Source: CAD feature listing. Evaluate the final solid. Frame: model axes, mm. Face numbers are marked on the shaded views. Give positions to 0.01 mm unless a question says otherwise; leave off trailing zeros. Loops run counter-clockwise (first coordinate to the right, second up) from the corner with the lowest first, then second, coordinate; pieces in that order, holes last. Notation, with made-up numbers: M -17.75,-13 L 12.25,-13 A17 cw 12.25,19 Z; hole C 85.5,50.5 d2. An arc over 180 degrees is marked long. Answer in a Markdown table with one row per item.
```python
from build123d import *

# Parameters (mm, degrees)
SKETCH1_R           = 37
BOSS_EXTRUDE1_DEPTH = 3.158172797
SKETCH13_W          = 7.575673387
SKETCH13_H          = 3.158172797
SKETCH13_W_2        = 7.5
BOSS_EXTRUDE2_DEPTH = 60
CIRPATTERN1_COUNT   = 4
SKETCH2_R           = 35
SKETCH2_R_2         = 6.35
CUT_EXTRUDE1_DEPTH  = 1
SKETCH17_R          = 2
CUT_EXTRUDE2_DEPTH  = 10
SKETCH19_R          = 1.5
CUT_EXTRUDE3_DEPTH  = 10
CIRPATTERN2_COUNT   = 4


with BuildPart() as part:
    # Sketch1 → Boss-Extrude1 (new body)
    with BuildSketch(Plane(origin=(0, 0, 0), x_dir=(1, 0, 0), z_dir=(0, 1, 0))):
        Circle(SKETCH1_R)
    extrude(amount=BOSS_EXTRUDE1_DEPTH)

    # Sketch13 → Boss-Extrude2 (add)
    with BuildSketch(Plane.XY):
        with Locations((3.787836694, 1.579086399)):
            Rectangle(SKETCH13_W, SKETCH13_H)
        with Locations((-3.75, 1.579086399)):
            Rectangle(SKETCH13_W_2, SKETCH13_H)
    boss_extrude2 = extrude(amount=BOSS_EXTRUDE2_DEPTH)

    # CirPattern1: Boss-Extrude2 ×4 about axis
    cirpattern1_axis = Axis((0, 0, 0), (0, 1, 0))
    for i in range(1, CIRPATTERN1_COUNT):
        add(boss_extrude2.rotate(cirpattern1_axis, i * 360 / CIRPATTERN1_COUNT))

    # Sketch2 → Cut-Extrude1 (cut)
    with BuildSketch(Plane(origin=(0, 3.158172797, 0), x_dir=(1, 0, 0), z_dir=(0, 1, 0))):
        Circle(SKETCH2_R)
        Circle(SKETCH2_R_2, mode=Mode.SUBTRACT)
    extrude(amount=-CUT_EXTRUDE1_DEPTH, mode=Mode.SUBTRACT)

    # Sketch17 → Cut-Extrude2 (cut)
    with BuildSketch(Plane(origin=(0, 3.158172797, 0), x_dir=(1, 0, 0), z_dir=(0, 1, 0))):
        Circle(SKETCH17_R)
    extrude(amount=-CUT_EXTRUDE2_DEPTH, mode=Mode.SUBTRACT)

    # Sketch19 → Cut-Extrude3 (cut)
    with BuildSketch(Plane(origin=(0, 3.158172797, 0), x_dir=(1, 0, 0), z_dir=(0, 1, 0))):
        with Locations((0, 25)):
            Circle(SKETCH19_R)
    cut_extrude3 = extrude(amount=-CUT_EXTRUDE3_DEPTH, mode=Mode.SUBTRACT)

    # CirPattern2: Cut-Extrude3 ×4 about axis
    cirpattern2_axis = Axis((0, 0, 0), (0, 1, 0))
    for i in range(1, CIRPATTERN2_COUNT):
        add(cut_extrude3.rotate(cirpattern2_axis, i * 360 / CIRPATTERN2_COUNT), mode=Mode.SUBTRACT)


solid = part.part
```
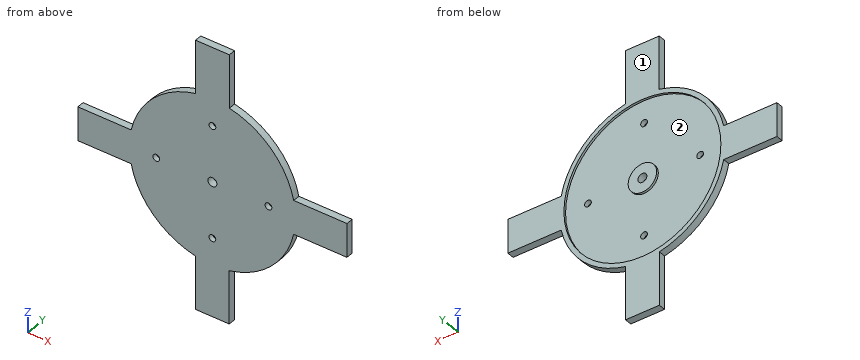
1) Pull-direction query (X, two-part tool) for the marked faces 1 and 2; classes: released by +X, released by -X, zero draft, split by the parting line, or undercut.
Reply:
| item | result |
|---|---|
| face 1 | zero draft |
| face 2 | undercut |
2) Section C-C, the plane x = 0. Return loops of the section in (y, z).
Reply:
| item | result |
|---|---|
| outline | M 0,-60 L 3.16,-60 L 3.16,-35 L 2.16,-35 L 2.16,-26.5 L 0,-26.5 Z; M 0,-23.5 L 2.16,-23.5 L 2.16,-6.35 L 3.16,-6.35 L 3.16,-2 L 0,-2 Z; M 0,2 L 3.16,2 L 3.16,6.35 L 2.16,6.35 L 2.16,23.5 L 0,23.5 Z; M 0,26.5 L 2.16,26.5 L 2.16,35 L 3.16,35 L 3.16,60 L 0,60 Z |
3) Section D-D, the plane z = -25. Return loops of the section in (x, y).
Reply:
| item | result |
|---|---|
| outline | M -27.28,0 L -1.5,0 L -1.5,2.16 L -24.49,2.16 L -24.49,3.16 L -27.28,3.16 Z; M 1.5,0 L 27.28,0 L 27.28,3.16 L 24.49,3.16 L 24.49,2.16 L 1.5,2.16 Z |
4) Pin query (flat end, axial travel): pin 1 Ø0.9 at (y, z) = (1, 51) entering from +X; pin 2 Ø3.5 at (x, z) = (0, -25) entering from +Y; pin 3 Ø0.9 at (x, y) = (-54, 2.5) entering from +Z. Return the tip coordinate at first contact, or that it passes through.
Reply:
| item | result |
|---|---|
| pin 1 | stops at x = 7.58 |
| pin 2 | stops at y = 2.16 |
| pin 3 | stops at z = 7.58 |
5) Section A-A, the plane z = 0. Return loops of the section in (x, y), then the cut area to 3 significant figures.
Reply:
| item | result |
|---|---|
| outline | M -60,0 L -26.5,0 L -26.5,2.16 L -35,2.16 L -35,3.16 L -60,3.16 Z; M -23.5,0 L -2,0 L -2,3.16 L -6.35,3.16 L -6.35,2.16 L -23.5,2.16 Z; M 2,0 L 23.5,0 L 23.5,2.16 L 6.35,2.16 L 6.35,3.16 L 2,3.16 Z; M 26.5,0 L 60,0 L 60,3.16 L 35,3.16 L 35,2.16 L 26.5,2.16 Z |
| area | 296 mm² |
6) Material intervals for L1, parallel to X at y = 2.6, z = 0; L2, parallel to Z at x = 0, y = 1.85, sorted ascending.
Reply:
| item | result |
|---|---|
| L1 | x = -60 to -35, -6.35 to -2, 2 to 6.35, 35 to 60 |
| L2 | z = -60 to -26.5, -23.5 to -2, 2 to 23.5, 26.5 to 60 |
7) Section B-B, the plane y = 1.1. Return loops of the section in (x, z).
Reply:
| item | result |
|---|---|
| outline | M -60,-7.5 L -36.23,-7.5 A37 ccw -7.58,-36.22 L -7.58,-60 L 7.5,-60 L 7.5,-36.23 A37 ccw 36.22,-7.58 L 60,-7.58 L 60,7.5 L 36.23,7.5 A37 ccw 7.58,36.22 L 7.58,60 L -7.5,60 L -7.5,36.23 A37 ccw -36.22,7.58 L -60,7.58 Z; hole C -25,0 d3; hole C 0,0 d4; hole C 0,-25 d3; hole C 0,25 d3; hole C 25,0 d3 |
